The figure shows three views and two pictorial views of one solid part (mm, origin at its lowest corner). Answer the questions. A direction names the side the tool comes from. Give positions to 0.01 mm unless a question says otherwise; leave off trailing zeros. Loops run counter-clockwise (first coordinate to the right, second up) from the corner with the lowest first, then second, coordinate; pieces in that order, holes last. Notation, with made-up numbers: (62.25, 17.5) -> (82.25, 17.5) arc R8 cw to (82.25, 29.5) -> close; hole circle Ø8 at (46, 34). An arc over 180 degrees is marked (long way). One line per item, written item: value. Start each with the question number.
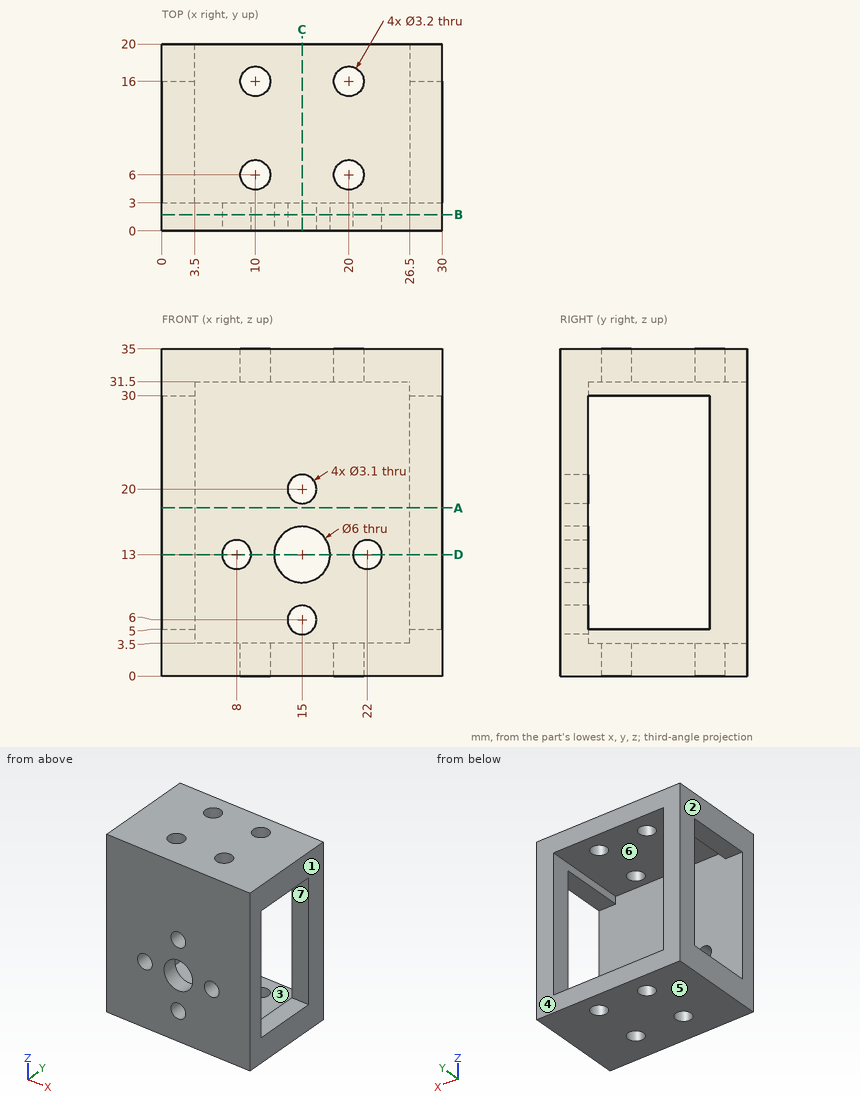
Item 1: For the marked faces 5, 6 and 7, determine the directions among +Z, -Z, +X, -X, +Y, -Y from which every point of the face is accessible in a straight line to the end or side of a thin tool.
Item 2: Consider L1, parallel to Y at x = 20, z = 0.8; L2, parallel to Z at x = 12.5, y = 16; L3, parallel to Z at x = 28.5, y = 14.75. Determine where each line is inside the solid, lowest interval first. Write a range as [from, to].
Item 3: Section C-C, the plane x = 15 is taken. Determine the outline of the cut face in (y, z), plus the area to 3 significant figures.
Item 4: Determine the mould class of the marked faces 1, 2, 3 and 4 for opening direction X: pulls with the +X half, pulls with the -X half, needs draft (parallel to the pull), parting line crosses it, or undercut.
Item 5: Section A-A, the plane z = 18 is taken. Determine the outline of the cut face in (x, y).
Item 6: Section B-B, the plane y = 1.75 is taken. Determine the outline of the cut face in (x, z).
Item 7: Section D-D, the plane z = 13 is taken. Determine the outline of the cut face in (x, y), plus the area to 3 significant figures.
Computed values:
1. face 5: -Z, +X, -X, +Y, -Y
1. face 6: +Y
1. face 7: +X, -X
2. L1: [0, 4.4], [7.6, 14.4], [17.6, 20]
2. L2: [0, 3.5], [31.5, 35]
2. L3: [0, 5], [30, 35]
3. outline: (0, 0) -> (20, 0) -> (20, 3.5) -> (3, 3.5) -> (3, 4.45) -> (0, 4.45) -> close; (0, 7.55) -> (3, 7.55) -> (3, 10) -> (0, 10) -> close; (0, 16) -> (3, 16) -> (3, 18.45) -> (0, 18.45) -> close; (0, 21.55) -> (3, 21.55) -> (3, 31.5) -> (20, 31.5) -> (20, 35) -> (0, 35) -> close
3. area: 187 mm²
4. face 1: pulls with the +X half
4. face 2: pulls with the -X half
4. face 3: undercut
4. face 4: needs draft
5. outline: (0, 0) -> (30, 0) -> (30, 3) -> (0, 3) -> close; (0, 16) -> (3.5, 16) -> (3.5, 20) -> (0, 20) -> close; (26.5, 16) -> (30, 16) -> (30, 20) -> (26.5, 20) -> close
6. outline: (0, 0) -> (30, 0) -> (30, 35) -> (0, 35) -> close; hole circle Ø3.1 at (8, 13); hole circle Ø6 at (15, 13); hole circle Ø3.1 at (15, 6); hole circle Ø3.1 at (15, 20); hole circle Ø3.1 at (22, 13)
7. outline: (0, 0) -> (6.45, 0) -> (6.45, 3) -> (0, 3) -> close; (0, 16) -> (3.5, 16) -> (3.5, 20) -> (0, 20) -> close; (9.55, 0) -> (12, 0) -> (12, 3) -> (9.55, 3) -> close; (18, 0) -> (20.45, 0) -> (20.45, 3) -> (18, 3) -> close; (23.55, 0) -> (30, 0) -> (30, 3) -> (23.55, 3) -> close; (26.5, 16) -> (30, 16) -> (30, 20) -> (26.5, 20) -> close
7. area: 81.4 mm²
